The listing builds one solid part. Answer for the finished solid, in the listing's coordinates (mm). Face numbers are marked on the shaded views. A direction names the side the tool comes from. Coordinates: 2 decimals unless noted, no trailing zeros. Loops run counter-clockwise (first coordinate to the right, second up) from the corner with the lowest first, then second, coordinate; pieces in that order, holes last. Notation, with made-up numbers: M 29,46 L 67,46 A13 ccw 67,51 Z; hole C 53.5,24 d8. An arc over 180 degrees is marked long. Answer as CSV lines item,"result". Start each with the question number.
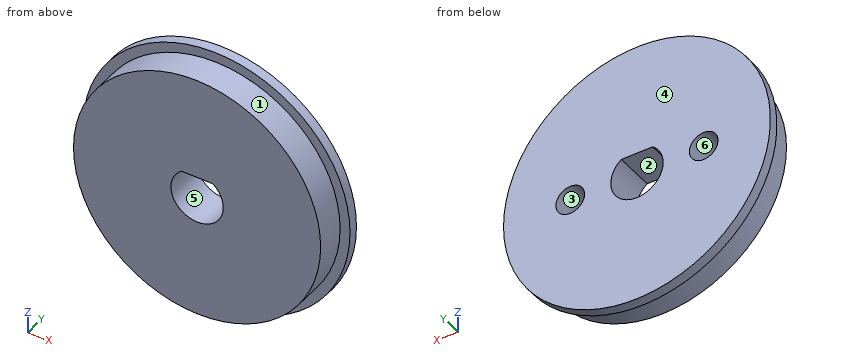
Autodesk Inventor part; units mm, degrees
ref_plane "YZ Plane" through (0, 0, 0) normal (1, 0, 0) x (0, 1, 0)
ref_plane "XZ Plane" through (0, 0, 0) normal (0, 1, 0) x (-1, 0, 0)
ref_plane "XY Plane" through (0, 0, 0) normal (0, 0, 1) x (1, 0, 0)
sketch "Szkic1" plane through (0, 0, 0) normal (0, 1, 0) x (-1, 0, 0)
  circle A0 centre (0, 0) radius 12.5
  dimension "d0" = 25
extrude "Wyciągnięcie proste1" add sketch "Szkic1" along normal blind 3
sketch "Szkic6" plane through (0, 3, 0) normal (0, 1, 0) x (1, 0, 0)
  circle A0 centre (0, 0) radius 13.5
  dimension "d13" = 27
extrude "Wyciągnięcie proste5" add sketch "Szkic6" along normal blind 1
sketch "Szkic7" plane through (0, 4, 0) normal (0, 1, 0) x (1, 0, 0)
  point P0 (0, 0)
  point P1 (-6.75, 0)
  dimension "d16" = 6.75
hole "Otwór1" at (-6.75, 4, 0) direction (0, -1, 0) diameter 2.9 depth 3
pattern_circular "Szyk kołowy1" count 2 over 360 about axis through (0, 3, 0) along (0, 1, 0) of "Otwór1"
sketch "Szkic8" plane through (0, 0, 0) normal (0, -1, 0) x (1, 0, 0)
  arc A0 (-1.59, 2.12) -> (1.59, 2.12) centre (0, 0) ccw
  line L0 (1.59, 2.12) -> (-1.59, 2.12)
  dimension "d27" = 5.3
extrude "Wyciągnięcie proste6" cut sketch "Szkic8" against normal through all
properties part number "_Drukowanie 3D"
Item 1: Section C-C on y = 1.4 is taken. Determine the outline of the cut face in (x, z), then the cut area to 3 significant figures.
Item 2: Consider line 1 (X direction, y = 1.2, z = -0.25); line 2 (Z direction, x = 0, y = 1.7); line 3 (Y direction, x = 3.5, z = 12.25). Determine where each line is inside the solid, lowest interval first.
Item 3: For the marked faces 5 and 6, determine the directions among +Z, -Z, +X, -X, +Y, -Y from which every point of the face is accessible in a straight line to the end or side of a thin tool.
Item 4: Each of these flat-tipped pins is pushed along its axis until it touches: P1, Ø1.7, axis at x = -6.75, z = 0, coming from the -Y side; P2, Ø4, axis at x = 0, z = 0, coming from the +Y side; P3, Ø1.7, axis at x = 6.75, z = 0, coming from the +Y side; P4, Ø1.5, axis at y = 1.5, z = 1, coming from the +X side. Where does it stop, or does it pass through?
Item 5: Section B-B on x = 0 is taken. Determine the outline of the cut face in (y, z).
Item 6: Section A-A on z = 0 is taken. Determine the outline of the cut face in (x, y).
Item 7: For a pull along X with two mould halves and no side action, classify the marked faces 1, 2, 3 and 4 as pulls with the +X half, pulls with the -X half, needs draft (parallel to the pull), parting line crosses it, or undercut.
Item 8: Section D-D on x = 4 is taken. Determine the outline of the cut face in (y, z), then the cut area to 3 significant figures.
Results are:
1,outline,"C 0,0 d25; hole C -6.75,0 d2.9; hole M -1.59,2.12 A2.65 ccw long 1.59,2.12 Z; hole C 6.75,0 d2.9"
1,area,"457 mm²"
2,line 1,"-12.5 to -8.18, -5.32 to -2.64, 2.64 to 5.32, 8.18 to 12.5"
2,line 2,"-12.5 to -2.65, 2.12 to 12.5"
2,line 3,"3 to 4"
3,face 5,"+Y, -Y"
3,face 6,"+Y"
4,P1,"y = 0"
4,P2,"through"
4,P3,"y = 1"
4,P4,"x = 12.5"
5,outline,"M 0,-12.5 L 3,-12.5 L 3,-13.5 L 4,-13.5 L 4,-2.65 L 0,-2.65 Z; M 0,2.12 L 4,2.12 L 4,13.5 L 3,13.5 L 3,12.5 L 0,12.5 Z"
6,outline,"M -13.5,3 L -12.5,3 L -12.5,0 L -2.65,0 L -2.65,4 L -5.3,4 L -5.3,1 L -8.2,1 L -8.2,4 L -13.5,4 Z; M 2.65,0 L 12.5,0 L 12.5,3 L 13.5,3 L 13.5,4 L 8.2,4 L 8.2,1 L 5.3,1 L 5.3,4 L 2.65,4 Z"
7,face 1,"parting line crosses it"
7,face 2,"undercut"
7,face 3,"undercut"
7,face 4,"needs draft"
8,outline,"M 0,-11.84 L 3,-11.84 L 3,-12.89 L 4,-12.89 L 4,12.89 L 3,12.89 L 3,11.84 L 0,11.84 Z"
8,area,"96.8 mm²"
